from build123d import *

# Parameters (mm, degrees)
BOSS_EXTRU_1_DEPTH      = 1.5
ESQUISSE7_R             = 1.5
ENL_V_MAT_EXTRU_5_DEPTH = 230.841793415
ESQUISSE8_R             = 19.627416998
ESQUISSE8_R_2           = 1.5
ENL_V_MAT_EXTRU_6_DEPTH = 230.841793415
ESQUISSE9_R             = 1.5
ESQUISSE9_R_2           = 2
ENL_V_MAT_EXTRU_7_DEPTH = 230.841793415
ENL_V_MAT_EXTRU_8_DEPTH = 230.841793415
CONG_1_R                = 1
ESQUISSE11_R            = 1.5
ENL_V_MAT_EXTRU_9_DEPTH = 230.841793415


with BuildPart() as part:
    # Esquisse1 → Boss.-Extru.1 (new body)
    with BuildSketch(Plane(origin=(0, 0, 0), x_dir=(1, 0, 0), z_dir=(0, 1, 0))):
        with BuildLine():
            Line((0, 49), (165, 49))
            Line((165, 49), (165, -55.235857919))
            ThreePointArc((165, -55.235857919), (127.908511428, -117.963607542), (68.381283989, -160))
            Line((68.381283989, -160), (0, -160))
            Line((0, -160), (0, 49))
        make_face()
    extrude(amount=BOSS_EXTRU_1_DEPTH)

    # Symétrie1: part across plane


with BuildPart() as part_1:
    add(part.part)
    add(part.part.mirror(Plane(origin=(0, 1.5, -49), x_dir=(0, 0, 1), z_dir=(1, 0, 0))))

    # Esquisse7 → Enlèv. mat.-Extru.5 (cut, through all)
    with BuildSketch(Plane(origin=(0, 1.5, 0), x_dir=(1, 0, 0), z_dir=(0, 1, 0))):
        with Locations(Location((-157, -43, 0), (0, 0, 270))):
            Circle(ESQUISSE7_R)
        with Locations(Location((157, -43, 0), (0, 0, 270))):
            Circle(ESQUISSE7_R)
        with Locations(Location((157, 43, 0), (0, 0, 270))):
            Circle(ESQUISSE7_R)
        with Locations(Location((-157, 43, 0), (0, 0, 270))):
            Circle(ESQUISSE7_R)
        with Locations(Location((-114, 43, 0), (0, 0, 270))):
            Circle(ESQUISSE7_R)
        with Locations(Location((-90, 43, 0), (0, 0, 270))):
            Circle(ESQUISSE7_R)
        with Locations(Location((90, 43, 0), (0, 0, 90))):
            Circle(ESQUISSE7_R)
        with Locations(Location((114, 43, 0), (0, 0, 90))):
            Circle(ESQUISSE7_R)
    extrude(amount=-ENL_V_MAT_EXTRU_5_DEPTH, mode=Mode.SUBTRACT)

    # Esquisse8 → Enlèv. mat.-Extru.6 (cut, through all)
    with BuildSketch(Plane(origin=(0, 1.5, 0), x_dir=(1, 0, 0), z_dir=(0, 1, 0))):
        with Locations(Location((-90, 2.5, 0), (0, 0, 270))):
            Circle(ESQUISSE8_R)
        with Locations(Location((-112.627416998, 2.5, 0), (0, 0, 270))):
            Circle(ESQUISSE8_R_2)
        with Locations(Location((-67.372583002, 2.5, 0), (0, 0, 270))):
            Circle(ESQUISSE8_R_2)
        with Locations(Location((112.627416998, 2.5, 0), (0, 0, 90))):
            Circle(ESQUISSE8_R_2)
        with Locations(Location((67.372583002, 2.5, 0), (0, 0, 90))):
            Circle(ESQUISSE8_R_2)
        with Locations(Location((90, 2.5, 0), (0, 0, 90))):
            Circle(ESQUISSE8_R)
    extrude(amount=-ENL_V_MAT_EXTRU_6_DEPTH, mode=Mode.SUBTRACT)

    # Esquisse9 → Enlèv. mat.-Extru.7 (cut, through all)
    with BuildSketch(Plane(origin=(0, 1.5, 0), x_dir=(1, 0, 0), z_dir=(0, 1, 0))):
        with Locations(Location((27.5, 32.5, 0), (0, 0, 270))):
            Circle(ESQUISSE9_R)
        with Locations(Location((-13, -30, 0), (0, 0, 270))):
            Circle(ESQUISSE9_R)
        with Locations(Location((35, -20, 0), (0, 0, 270))):
            Circle(ESQUISSE9_R)
        with Locations(Location((-27.5, 32.5, 0), (0, 0, 90))):
            Circle(ESQUISSE9_R)
        with Locations(Location((0, 0, 0), (0, 0, 270))):
            Circle(ESQUISSE9_R_2)
        with Locations(Location((-35, -20, 0), (0, 0, 90))):
            Circle(ESQUISSE9_R)
        with Locations(Location((13, -30, 0), (0, 0, 90))):
            Circle(ESQUISSE9_R)
        with BuildLine():
            Line((4, 49), (4, 42))
            ThreePointArc((4, 42), (0, 38), (-4, 42))
            Line((-4, 42), (-4, 49))
            ThreePointArc((-4, 49), (0, 53), (4, 49))
        make_face()
    extrude(amount=-ENL_V_MAT_EXTRU_7_DEPTH, mode=Mode.SUBTRACT)

    # Esquisse10 → Enlèv. mat.-Extru.8 (cut, through all)
    with BuildSketch(Plane(origin=(0, 1.5, 0), x_dir=(1, 0, 0), z_dir=(0, 1, 0))):
        with BuildLine():
            Line((43, -73), (43, -150))
            ThreePointArc((43, -150), (40, -153), (37, -150))
            Line((37, -150), (37, -73))
            ThreePointArc((37, -73), (40, -70), (43, -73))
        make_face()
    extrude(amount=-ENL_V_MAT_EXTRU_8_DEPTH, mode=Mode.SUBTRACT)

    # Congé1
    cong_1_edges = [part_1.edges().sort_by_distance(p)[0] for p in [
        (-165, 0.75, -49),
        (165, 0.75, -49),
    ]]
    fillet(cong_1_edges, radius=CONG_1_R)

    # Esquisse11 → Enlèv. mat.-Extru.9 (cut, through all)
    with BuildSketch(Plane(origin=(0, 1.5, 0), x_dir=(1, 0, 0), z_dir=(0, 1, 0))):
        with Locations(Location((-150.869773386, -69.240966765, 0), (0, 0, 270))):
            Circle(ESQUISSE11_R)
        with Locations(Location((-116.399964779, -118.351375994, 0), (0, 0, 270))):
            Circle(ESQUISSE11_R)
        with Locations(Location((-66.72330927, -152, 0), (0, 0, 270))):
            Circle(ESQUISSE11_R)
        with Locations(Location((66.72330927, -152, 0), (0, 0, 90))):
            Circle(ESQUISSE11_R)
        with Locations(Location((116.399964779, -118.351375994, 0), (0, 0, 90))):
            Circle(ESQUISSE11_R)
        with Locations(Location((150.869773386, -69.240966765, 0), (0, 0, 90))):
            Circle(ESQUISSE11_R)
        with Locations(Location((-15, -152, 0), (0, 0, 270))):
            Circle(ESQUISSE11_R)
        with Locations(Location((15, -152, 0), (0, 0, 90))):
            Circle(ESQUISSE11_R)
    extrude(amount=-ENL_V_MAT_EXTRU_9_DEPTH, mode=Mode.SUBTRACT)


solid = part_1.part
Design review of the part built by this model. Coordinates are the model's own, in mm. Round coordinates to 2 decimals unless told otherwise and drop trailing zeros. Write each loop counter-clockwise with the first axis right and the second up, starting at its lowest first coordinate (ties: lowest second). Pieces come first, ordered by that corner, then holes.
Item 1: Draft analysis for pull direction X (two halves, no side actions). For faces 1 (the flat face through (-2, 1.5, 54)), 2 (the cylindrical face through (-109.16, 0.76, -6.75)), 3 (the cylindrical face through (-128.6, 0.74, 117.21)), state which applies: released by +X, released by -X, zero draft, split by the parting line, or undercut.
Item 2: Consider section A-A on z = 135.5. Give the boundary of the cut face in (x, y).
Item 3: For pin 1 Ø1.8 at (x, z) = (-15, 152) entering from +Y, flat-tipped, find the tip position at first contact; note if it passes through.
Item 4: Consider section B-B on x = -75. Give the boundary of the cut face in (y, z), and give its area (3 significant figures).
Item 5: Consider section D-D on y = 0.8. Count the separate pieces of the cut face and the enclosed holes in it, and give its area (3 significant figures).
Item 6: Consider section C-C on z = 6.5. Give the boundary of the cut face in (x, y), and give its area (3 significant figures).
Item 7: Wall thickness on L1, parallel to X at y = 0.75, z = 43; L2, parallel to X at y = 0.7, z = 20; L3, parallel to Z at x = 90, y = 0.7: over which ranges is each line inside the solid? List them lowest first.
Check values:
1. face 1: zero draft
1. face 2: undercut
1. face 3: released by -X
2. outline: (-109.16, 0) - (37, 0) - (37, 1.5) - (-109.16, 1.5) - close; (43, 0) - (109.16, 0) - (109.16, 1.5) - (43, 1.5) - close
3. pin 1: passes through
4. outline: (0, -49) - (1.5, -49) - (1.5, -15.16) - (0, -15.16) - close; (0, 10.16) - (1.5, 10.16) - (1.5, 157.01) - (0, 157.01) - close
4. area: 271 mm2
5. separate pieces: 1
5. enclosed holes: 30
5. area: 58,600 mm2
6. outline: (-165, 0) - (-107.44, 0) - (-107.44, 1.5) - (-165, 1.5) - close; (-72.56, 0) - (72.56, 0) - (72.56, 1.5) - (-72.56, 1.5) - close; (107.44, 0) - (165, 0) - (165, 1.5) - (107.44, 1.5) - close
6. area: 390 mm2
7. L1: x = -165 to -158.5, -155.5 to 155.5, 158.5 to 165
7. L2: x = -165 to -36.5, -33.5 to 33.5, 36.5 to 165
7. L3: z = -49 to -44.5, -41.5 to -22.13, 17.13 to 148.92
